Verification items for the finished model (mm, model axes). A direction names the side the tool comes from. Coordinates: 2 decimals unless noted, no trailing zeros. Order: outer loops, then holes, each group sorted by start corner. A loop starts at its lowest first (then second) coordinate and runs counter-clockwise, first axis right, second up. Notation, with made-up numbers: M 43,64.5 L 102,64.5 A27 ccw 102,100.5 Z; hole C -11,-21.5 d2. An arc over 180 degrees is marked long. Answer as a JSON object with one key per item and string values. Group by question number.
(1) Cross-section at B-B (z = 2.5). Enter the section's corners in (x, y) (3 decimals), plus the area to 3 significant figures.
(2) Material ranges on line 1 (X direction, y = -79, z = 10); line 2 (Z direction, x = 505, y = -89.5); line 3 (Z direction, x = 301.5, y = -87.5), recorded low to high.
(3) Cross-section at A-A (x = 376). Enter the section's corners in (y, z), plus the area to 3 significant figures.
(4) Access from +Z, -Z, +X, -X, +Y, -Y to the whole of each face (thin tool, end or side, straight path). Record for faces 1 (the face through (299, -79, 27.432)), 2 (the face through (505.89, -83.85, -17.12)), 3 (the face through (515.77, -79, -16)), 4 (the face through (504.4, -83.2, -12.7)).
(5) Cross-section at C-C (z = 17). Enter the section's corners in (x, y).
(6) Gauge pin test, flat ends, axial feed: pin 1 Ø15 at (x, y) = (505, -81) entering from +Z; pin 2 Ø5 at (y, z) = (-77, -4) entering from -X; pin 3 Ø3 at (y, z) = (-78, -16.5) entering from +X; pin 4 Ø6 at (x, z) = (478.5, 14.5) entering from -Y. Record the tip position at first contact, or that the pin passes through.
(7) Mould release check, pull along Y, two halves, no side actions. Record for faces 5 (the face through (492, -66.361, -9)), 6 (the face through (491, -91.761, -9)), 7 (the face through (500.253, -74.271, -17.118)), 8 (the face through (317.699, -78.883, 21.317)): released by +Y, released by -Y, zero draft, split by the parting line, or undercut.
from build123d import *

# Parameters (mm, degrees)
SKETCH1_R            = 3.175
BOSS_EXTRUDE1_DEPTH  = 12.7
BOSS_EXTRUDE8_DEPTH  = 19.05
CUT_EXTRUDE3_DEPTH   = 41.148
BOSS_EXTRUDE9_DEPTH  = 25.4
BOSS_EXTRUDE11_DEPTH = 19.05
SKETCH10_W           = 19.05
SKETCH10_H           = 12.794581221
CUT_EXTRUDE5_DEPTH   = 25.4
BOSS_EXTRUDE12_DEPTH = 2.54
CUT_EXTRUDE6_DEPTH   = 25.4


with BuildPart() as part:
    # Sketch1 → Boss-Extrude1 (new body)
    with BuildSketch(Plane.XY):
        with BuildLine():
            Line((299.870251741, -63.185614448), (503.070251741, -63.185614448))
            ThreePointArc((503.070251741, -63.185614448), (518.945251741, -79.060614448), (503.070251741, -94.935614448))
            Line((503.070251741, -94.935614448), (299.870251741, -94.935614448))
            ThreePointArc((299.870251741, -94.935614448), (283.995251741, -79.060614448), (299.870251741, -63.185614448))
        make_face()
        with Locations((299.870251741, -79.060614448)):
            Circle(SKETCH1_R, mode=Mode.SUBTRACT)
        with Locations((503.070251741, -79.060614448)):
            Circle(SKETCH1_R, mode=Mode.SUBTRACT)
    extrude(amount=BOSS_EXTRUDE1_DEPTH)

    # Sketch7 → Boss-Extrude8 (add)
    with BuildSketch(Plane.XY.offset(12.7)):
        with BuildLine():
            Line((310.030251741, -66.360614448), (312.570251741, -66.360614448))
            Line((312.570251741, -66.360614448), (322.730251741, -66.360614448))
            Line((322.730251741, -66.360614448), (322.730251741, -91.760614448))
            Line((322.730251741, -91.760614448), (310.030251741, -91.760614448))
            Line((310.030251741, -91.760614448), (289.710251741, -91.760614448))
            ThreePointArc((289.710251741, -91.760614448), (287.914200517, -91.016665672), (287.170251741, -89.220614448))
            Line((287.170251741, -89.220614448), (287.170251741, -68.900614448))
            ThreePointArc((287.170251741, -68.900614448), (287.914200517, -67.104563223), (289.710251741, -66.360614448))
            Line((289.710251741, -66.360614448), (310.030251741, -66.360614448))
        make_face()
    extrude(amount=BOSS_EXTRUDE8_DEPTH)

    # Sketch8 → Cut-Extrude3 (cut)
    with BuildSketch(Plane(origin=(0, -66.360614448, 0), x_dir=(1, 0, 0), z_dir=(0, 1, 0))):
        with BuildLine():
            Line((287.170251741, -12.7), (317.904251741, -12.7))
            ThreePointArc((317.904251741, -12.7), (317.648023156, -21.431345807), (311.300251741, -27.432))
            Line((311.300251741, -27.432), (287.170251741, -27.432))
            Line((287.170251741, -27.432), (287.170251741, -12.7))
        make_face()
    extrude(amount=-CUT_EXTRUDE3_DEPTH, mode=Mode.SUBTRACT)

    # Sketch9 → Boss-Extrude9 (add)
    with BuildSketch(Plane(origin=(0, -66.360614448, 0), x_dir=(1, 0, 0), z_dir=(0, 1, 0))):
        Polygon((322.730251741, -31.75), (349.936471269, -12.7), (322.730251741, -12.7), align=None)
    extrude(amount=-BOSS_EXTRUDE9_DEPTH)

    # Sketch2 → Boss-Extrude11 (add)
    with BuildSketch(Plane(origin=(0, 0, 0), x_dir=(-1, 0, 0), z_dir=(0, 0, -1))):
        with BuildLine():
            Line((-477.670251741, -66.360614448), (-477.670251741, -91.760614448))
            Line((-477.670251741, -91.760614448), (-513.230251741, -91.760614448))
            ThreePointArc((-513.230251741, -91.760614448), (-515.026302965, -91.016665672), (-515.770251741, -89.220614448))
            Line((-515.770251741, -89.220614448), (-515.770251741, -68.900614448))
            ThreePointArc((-515.770251741, -68.900614448), (-515.026302965, -67.104563223), (-513.230251741, -66.360614448))
            Line((-513.230251741, -66.360614448), (-477.670251741, -66.360614448))
        make_face()
        Polygon((-503.070251741, -72.644809581), (-508.626501741, -75.852712014), (-508.626501741, -82.268516881), (-503.070251741, -85.476419314), (-497.514001741, -82.268516881), (-497.514001741, -75.852712014), align=None, mode=Mode.SUBTRACT)
    extrude(amount=BOSS_EXTRUDE11_DEPTH)

    # Sketch10 → Cut-Extrude5 (cut)
    with BuildSketch(Plane.XZ.offset(91.760614448)):
        with Locations((506.245251741, -6.397290611)):
            Rectangle(SKETCH10_W, SKETCH10_H)
    extrude(amount=-CUT_EXTRUDE5_DEPTH, mode=Mode.SUBTRACT)

    # Sketch11 → Boss-Extrude12 (add)
    with BuildSketch(Plane(origin=(0, 0, -12.7), x_dir=(-1, 0, 0), z_dir=(0, 0, -1))):
        Polygon((-503.070251741, -72.644809581), (-508.626501741, -75.852712014), (-508.626501741, -82.268516881), (-503.070251741, -85.476419314), (-497.514001741, -82.268516881), (-497.514001741, -75.852712014), align=None)
        Polygon((-503.070251741, -74.661205396), (-506.880251741, -76.860909922), (-506.880251741, -81.260318973), (-503.070251741, -83.460023499), (-499.260251741, -81.260318973), (-499.260251741, -76.860909922), align=None, mode=Mode.SUBTRACT)
    extrude(amount=BOSS_EXTRUDE12_DEPTH)

    # Sketch12 → Cut-Extrude6 (cut)
    with BuildSketch(Plane(origin=(0, -66.360614448, 0), x_dir=(1, 0, 0), z_dir=(0, 1, 0))):
        with BuildLine():
            Line((477.670251741, 6.35), (477.670251741, 9.525))
            Line((477.670251741, 9.525), (477.670251741, 19.05))
            Line((477.670251741, 19.05), (486.490339075, 19.05))
            Line((486.490339075, 19.05), (490.370251741, 19.05))
            ThreePointArc((490.370251741, 19.05), (481.38999562, 15.330256121), (477.670251741, 6.35))
        make_face()
    extrude(amount=-CUT_EXTRUDE6_DEPTH, mode=Mode.SUBTRACT)


solid = part.part
Taken from the geometry:
{
 "1": {"outline": "M 299.87,-94.936 L 503.07,-94.936 A15.875 ccw 503.07,-63.186 L 299.87,-63.186 A15.875 ccw Z; hole C 299.87,-79.061 d6.35; hole C 503.07,-79.061 d6.35", "area": "7,180 mm²"},
 "2": {"line 1": "x = 284 to 296.7, 303.04 to 499.9, 506.24 to 518.95", "line 2": "z = -19.05 to -12.79, 0 to 12.7", "line 3": "z = 0 to 12.7, 27.43 to 31.75"},
 "3": {"outline": "M -94.94,0 L -63.19,0 L -63.19,12.7 L -94.94,12.7 Z", "area": "403 mm²"},
 "4": {"face 1": "-X, +Y, -Y", "face 2": "-Z", "face 3": "-Z, +X, +Y, -Y", "face 4": "+X, +Y, -Y"},
 "5": {"outline": "M 318.65,-91.76 L 343.8,-91.76 L 343.8,-66.36 L 318.65,-66.36 Z"},
 "6": {"pin 1": "stops at z = 12.7", "pin 2": "stops at x = 477.67", "pin 3": "stops at x = 515.77", "pin 4": "stops at y = -94.94"},
 "7": {"face 5": "released by +Y", "face 6": "released by -Y", "face 7": "undercut", "face 8": "zero draft"}
}
